Design review of the part built by this model. Coordinates are the model's own, in mm. Face numbers are marked on the shaded views. A direction names the side the tool comes from. Coordinates: 2 decimals unless noted, no trailing zeros. Write each loop counter-clockwise with the first axis right and the second up, starting at its lowest first coordinate (ties: lowest second). Pieces come first, ordered by that corner, then holes. Notation, with made-up numbers: (76.25, 85) - (134.25, 85) arc R27 ccw to (134.25, 113) - close; hole circle Ø6 at (-35.5, -39). An arc over 180 degrees is marked (long way). Use a Markdown table: item, result.
from build123d import *

# Parameters (mm, degrees)
F1_DEPTH  = 500
F3_DEPTH  = 25
F5_DEPTH  = 25
F6_W      = 3
F6_H      = 22
F7_DEPTH  = 25
F8_W      = 22
F8_H      = 3
F9_DEPTH  = 25
F11_DEPTH = 3
F12_R     = 1.5
F13_R     = 2.5
F14_DEPTH = 25
F16_DEPTH = 3
F17_R     = 1.5
F18_R     = 2.5
F19_DEPTH = 25
F20_W     = 3
F20_H     = 502.47
F21_DEPTH = 25
F23_DEPTH = 3
F24_R     = 5
F25_DEPTH = 25


with BuildPart() as f1:
    # F0 (on Front) → F1 (new body)
    with BuildSketch(Plane.XZ):
        Polygon((504.47, 0), (0, 0), (-81.595, -141.3266856436), (-78.9969237661, -142.8266856566), (1.7320508226, -3.0000000261), (506.5706226329, -3.0000000261), (679.2355833198, 471.3930805921), (919.3296938381, 513.7281501857), (918.8087493006, 516.6825734704), (677.0089017035, 474.0467364079), align=None)
    extrude(amount=F1_DEPTH)

    # F2 (on face) → F3 (cut)
    with BuildSketch(Plane(origin=(0, 0, 0), x_dir=(0, -1, 0), z_dir=(-0.8660254038, 0, 0.5))):
        with BuildLine():
            add(Edge.make_bspline(
                [(0, -163.19), (92.9037991034, -155.737461166), (273.0256641206, -141.2884805339), (425.9509699186, -80.7188457637), (500, -51.39)],
                knots=[0, 0, 0, 0, 0.5157830178, 1, 1, 1, 1], degree=3))
            Line((0, -163.19), (0, -174.6820956469))
            Line((0, -174.6820956469), (528.7734270096, -174.6820956469))
            Line((528.7734270096, -174.6820956469), (528.7734270096, -51.39))
            Line((528.7734270096, -51.39), (500, -51.39))
        make_face()
    extrude(amount=-F3_DEPTH, mode=Mode.SUBTRACT)

    # F4 (on face) → F5 (cut)
    with BuildSketch(Plane(origin=(-60.6524500815, 0, 343.9771374623), x_dir=(0.984807753, 0, 0.1736481777), z_dir=(-0.1736481777, 0, 0.984807753))):
        with BuildLine():
            Line((994.5709671621, -500), (994.5709671621, 0))
            add(Edge.make_bspline(
                [(994.5709671621, 0), (985.1762808521, -87.1032361942), (966.2104639681, -262.9456191283), (875.4987714572, -420.4933030834), (829.7209671621, -500)],
                knots=[0, 0, 0, 0, 0.4953483611, 1, 1, 1, 1], degree=3))
            Line((829.7209671621, -500), (994.5709671621, -500))
        make_face()
    extrude(amount=-F5_DEPTH, mode=Mode.SUBTRACT)

    # F6 (on face) → F7 (cut)
    with BuildSketch(Plane(origin=(0, 0, 0), x_dir=(0, -1, 0), z_dir=(-0.8660254038, 0, 0.5))):
        with Locations((498.5, -19)):
            Rectangle(F6_W, F6_H)
    extrude(amount=-F7_DEPTH, mode=Mode.SUBTRACT)

    # F8 (on face) → F9 (cut)
    with BuildSketch(Plane(origin=(-60.6524500815, 0, 343.9771374623), x_dir=(0.984807753, 0, 0.1736481777), z_dir=(-0.1736481777, 0, 0.984807753))):
        with Locations((788.6809671621, -498.5)):
            Rectangle(F8_W, F8_H)
    extrude(amount=-F9_DEPTH, mode=Mode.SUBTRACT)

    # F10 (on face) → F11 (join)
    with BuildSketch(Plane.XZ.offset(497)):
        Polygon((730.4443408179, 456.8646688183), (725.894758563, 482.6666319473), (706.1986035028, 479.1936683939), (710.7481857577, 453.391705265), align=None)
    extrude(amount=F11_DEPTH)

    # F12
    f12_edges = [f1.edges().sort_by_distance(p)[0] for p in [
        (716.046681, -500, 480.93015),
        (716.567626, -497, 477.975727),
    ]]
    fillet(f12_edges, radius=F12_R)

    # F13 (on face) → F14 (cut)
    with BuildSketch(Plane.XZ.offset(500)):
        with Locations((719.7280223994, 460.0522258067)):
            Circle(F13_R)
    extrude(amount=-F14_DEPTH, mode=Mode.SUBTRACT)

    # F15 (on face) → F16 (join)
    with BuildSketch(Plane.XZ.offset(497)):
        Polygon((-4.5, -7.7942286341), (-14.5, -25.1147367097), (8.0339810065, -38.1247367097), (18.0339810065, -20.8042286341), align=None)
    extrude(amount=F16_DEPTH)

    # F17
    f17_edges = [f1.edges().sort_by_distance(p)[0] for p in [
        (-9.5, -500, -16.454483),
        (-6.901924, -497, -17.954483),
    ]]
    fillet(f17_edges, radius=F17_R)

    # F18 (on face) → F19 (cut)
    with BuildSketch(Plane.XZ.offset(500)):
        with Locations((8.7038539875, -26.9644826719)):
            Circle(F18_R)
    extrude(amount=-F19_DEPTH, mode=Mode.SUBTRACT)

    # F20 (on face) → F21 (cut)
    with BuildSketch(Plane(origin=(445.4582201101, 0, -162.1335327293), x_dir=(0, -1, 0), z_dir=(-0.9396926208, 0, 0.3420201433))):
        with Locations((498.5, 424.7739017035)):
            Rectangle(F20_W, F20_H)
    extrude(amount=-F21_DEPTH, mode=Mode.SUBTRACT)

    # F22 (on face) → F23 (join)
    with BuildSketch(Plane.XZ.offset(497)):
        Polygon((679.1439393037, 471.1412907274), (676.3248614168, 472.1673511663), (505.1540402867, 1.8793852416), (507.9731181735, 0.8533248027), align=None)
        Polygon((681.9630171416, 470.1152303063), (679.1439393037, 471.1412907274), (507.9731181735, 0.8533248027), (518.281546199, -2.8986361607), (571.1954295904, 0.9396926208), (680.732997499, 236.8955152162), align=None)
    extrude(amount=F23_DEPTH)

    # F24 (on face) → F25 (cut)
    with BuildSketch(Plane.XZ.offset(500)):
        with Locations((588.350177503, 75.9943071688)):
            Circle(F24_R)
        with Locations((638.6515103983, 163.4973151683)):
            Circle(F24_R)
    extrude(amount=-F25_DEPTH, mode=Mode.SUBTRACT)

    # F26: F1 across face


with BuildPart() as f1_1:
    add(f1.part)
    add(f1.part.mirror(Plane(origin=(434.4998955086, 0, 160.5222009708), x_dir=(1, 0, 0), z_dir=(0, 1, 0))))


solid = f1_1.part
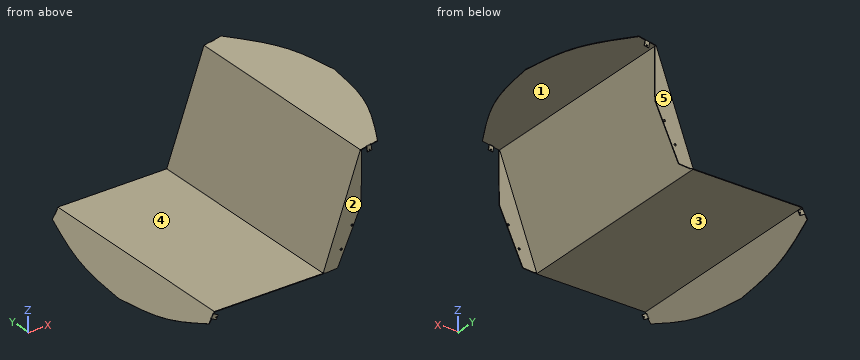
(1) For L1, parallel to Z at x = 20.5, y = 215; L2, parallel to Z at x = 815, y = 281.5; L3, parallel to X at y = 17, z = -6.5, list the stretches that pass through material, from the lowest coordinate up. Write a range as from..to.
Determined:
| item | result |
|---|---|
| L1 | -3..0 |
| L2 | 495.33..498.38 |
| L3 | -3.75..-0.29 |
(2) Take a section at B-B on x = 50.5. Write out the cut boundary in (y, z), and give its area (3 significant figures).
Determined:
| item | result |
|---|---|
| outline | (-500, -3) - (500, -3) - (500, 0) - (-500, 0) - close |
| area | 3,000 mm2 |
(3) For pin 1 (0.5 mm diameter, centred on x = 727, z = 480.5, fed in from -Y); pin 2 (8 mm diameter, centred on x = 8.7, z = -26.96, fed in from +Y); pin 3 (1 mm diameter, centred on x = 729, y = 15, fed in from +Z); pin 4 (4 mm diameter, centred on x = 201.5, y = -58, fed in from -Z), all flat-tipped, find the tip position at first contact; note any pin that passes through.
Determined:
| item | result |
|---|---|
| pin 1 | y = -497 |
| pin 2 | y = 500 |
| pin 3 | z = 483.3 |
| pin 4 | z = -3 |
(4) Take a section at A-A on z = 384.5. Write out the cut boundary in (x, y).
Determined:
| item | result |
|---|---|
| outline | (644.42, -500) - (681.51, -500) - (681.51, -497) - (647.61, -497) - (647.61, 497) - (681.51, 497) - (681.51, 500) - (644.42, 500) - close |
(5) Draft analysis for pull direction Y (two halves, no side actions). For the marked faces 1, 2 and 3, state which applies: +Y half, -Y half, draft (parallel to the pull), parting line (faces both ways), or undercut.
Determined:
| item | result |
|---|---|
| face 1 | undercut |
| face 2 | -Y half |
| face 3 | draft |
(6) Machinability: for the marked faces 4 and 5, which of the approach directions +Z, -Z, +X, -X, +Y, -Y give a long, thin tool a straight path to every point of the face, cutting with its end or side? Answer none if there is none.
Determined:
| item | result |
|---|---|
| face 4 | +Z, -X, +Y, -Y |
| face 5 | +Z, -Z, +X, -X, +Y |
